```python
from build123d import *

# Parameters (mm, degrees)
F1_DEPTH = 6.5
F2_R     = 2.5
F3_DEPTH = 8


with BuildPart() as f1:
    # F0 (on Top) → F1 (new body)
    with BuildSketch(Plane.XY):
        with BuildLine():
            ThreePointArc((-34.035903, 2.760554), (-20.149213, 6.068291), (-6.129181, 3.381293))
            ThreePointArc((-6.129181, 3.381293), (3.558859, -6.027813), (0, 7))
            ThreePointArc((0, 7), (-3.86946, 10.575604), (-8.367613, 13.318645))
            ThreePointArc((-8.367613, 13.318645), (-26.574298, 15.09931), (-41.627142, 4.703827))
            ThreePointArc((-41.627142, 4.703827), (-40.14959, -5.323154), (-34.035903, 2.760554))
        make_face()
        with BuildLine():
            ThreePointArc((-8.367613, 13.318645), (-3.86946, 10.575604), (0, 7))
            Line((0, 7), (12.165275, 12.823824))
            Line((12.165275, 12.823824), (12.165275, 16.940814))
            Line((12.165275, 16.940814), (8.897662, 19.496433))
            Line((8.897662, 19.496433), (-8.367613, 13.318645))
        make_face()
    extrude(amount=F1_DEPTH)

    # F2 (on face) → F3 (cut)
    with BuildSketch(Plane.XY.offset(6.5)):
        Circle(F2_R)
        with Locations((-38.786922, 0)):
            Circle(F2_R)
    extrude(amount=-F3_DEPTH, mode=Mode.SUBTRACT)


solid = f1.part
```
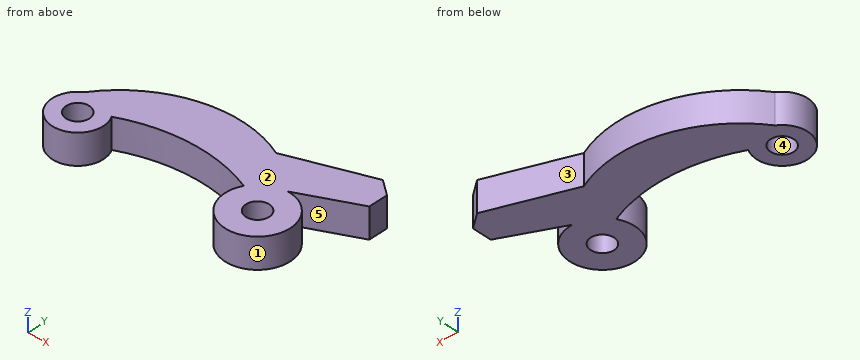
Geometry check sheet. Reference: the model listing, model coordinates, mm. Face numbers are marked on the shaded views. A direction names the side the tool comes from. Round coordinates to 2 decimals unless told otherwise and drop trailing zeros. Write each loop counter-clockwise with the first axis right and the second up, starting at its lowest first coordinate (ties: lowest second). Pieces come first, ordered by that corner, then holes. Notation, with made-up numbers: (3.25, -5.75) - (17.25, -5.75) arc R30 cw to (17.25, 26.25) - close; hole circle Ø8 at (-19, 54.5). An arc over 180 degrees is marked (long way). Write each question's results on one line, items separated by ' | '.
(1) Sectioned sample at A-A, the plane y = 0. Enter the section's corners in (x, z), plus the area to 3 significant figures.
Computed:
outline: (-44.28, 0) - (-41.29, 0) - (-41.29, 6.5) - (-44.28, 6.5) - close; (-36.29, 0) - (-33.29, 0) - (-33.29, 6.5) - (-36.29, 6.5) - close; (-7, 0) - (-2.5, 0) - (-2.5, 6.5) - (-7, 6.5) - close; (2.5, 0) - (7, 0) - (7, 6.5) - (2.5, 6.5) - close | area: 97.4 mm^2
(2) Draft check along Y on the marked faces 1, 2 and 3. Enter one of: pulls with the +Y half, pulls with the -Y half, needs draft (parallel to the pull), parting line crosses it, or undercut.
Computed:
face 1: undercut | face 2: needs draft | face 3: pulls with the +Y half
(3) Thickness scan on probe 1 along X at (y, z) = (0.25, 1.5); probe 2 along Y at (x, z) = (-40, 1); probe 3 along X at (y, z) = (-0.75, 5.25). Record the ranges inside material, lowest first. Write a range as from..to.
Computed:
probe 1: x = -44.28..-41.27, -36.3..-33.3, -7..-2.49, 2.49..7 | probe 2: y = -5.36..-2.19, 2.19..6.78 | probe 3: x = -44.23..-41.17, -36.4..-33.34, -6.96..-2.38, 2.38..6.96
(4) Sectioned sample at C-C, the plane z = 1.5. Enter the section's corners in (x, y), plus the area to 3 significant figures.
Computed:
outline: (-41.63, 4.7) arc R5.49 ccw (long way) to (-34.04, 2.76) arc R33.98 cw to (-6.13, 3.38) arc R7 ccw (long way) to (0, 7) - (12.17, 12.82) - (12.17, 16.94) - (8.9, 19.5) - (-8.37, 13.32) arc R26.61 ccw to start; hole circle Ø5 at (-38.79, 0); hole circle Ø5 at (0, 0) | area: 664 mm^2
(5) Set-up check for the marked faces 4 and 5: record each of +Z, -Z, +X, -X, +Y, -Y from which the full face is reachable in a straight line by a thin tool's end or side.
Computed:
face 4: +Z, -Z | face 5: +Z, -Z, +X
(6) Depth check by flat-ended pin: pin 1 Ø4 at (x, y) = (-38.79, 0) entering from -Z; pin 2 Ø3 at (x, z) = (-2, 5) entering from +Y; pin 3 Ø2 at (y, z) = (9, 0.5) entering from -X; pin 4 Ø3 at (y, z) = (9.5, 4.5) entering from +X. Enter the tip coordinate at first touch or a pass-through.
Computed:
pin 1: passes through | pin 2: stops at y = 16.13 | pin 3: stops at x = -38.87 | pin 4: stops at x = 8.36
(7) Sectioned sample at B-B, the plane x = 5. Enter the section's corners in (y, z), plus the area to 3 significant figures.
Computed:
outline: (-4.9, 0) - (4.9, 0) - (4.9, 6.5) - (-4.9, 6.5) - close; (9.39, 0) - (18.1, 0) - (18.1, 6.5) - (9.39, 6.5) - close | area: 120 mm^2
(8) Sectioned sample at D-D, the plane y = 9.25. Enter the section's corners in (x, z).
Computed:
outline: (-37.56, 0) - (4.7, 0) - (4.7, 6.5) - (-37.56, 6.5) - close
